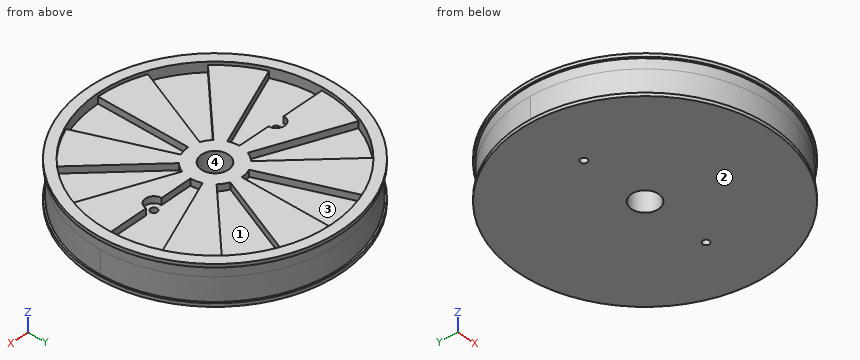
from build123d import *
from build123d.topology import SkipClean

# Parameters (mm, degrees)
CROQUIS1_R                 = 37.5
SALIENTE_EXTRUIR1_DEPTH    = 3.5
CROQUIS3_R                 = 38
SALIENTE_EXTRUIR2_DEPTH    = 1
SALIENTE_EXTRUIR4_START    = 1
CROQUIS5_R                 = 38
SALIENTE_EXTRUIR4_DEPTH    = 1
CROQUIS6_R                 = 4.05
CORTAR_EXTRUIR1_DEPTH      = 31
SALIENTE_EXTRUIR5_START    = 2
CROQUIS7_R                 = 8
CROQUIS7_R_2               = 4.05
SALIENTE_EXTRUIR5_DEPTH    = 2
SALIENTE_EXTRUIR7_START    = 2
SALIENTE_EXTRUIR7_DEPTH    = 2
SALIENTE_EXTRUIR8_START    = 3
CROQUIS10_R                = 38
CROQUIS10_R_2              = 35
SALIENTE_EXTRUIR8_DEPTH    = 3
CORTAR_EXTRUIR2_DEPTH      = 21
CORTAR_EXTRUIR2_DEPTH_BACK = 48
CROQUIS11_R                = 1
CROQUIS15_OUTSIDE_W        = 99.63
CROQUIS15_OUTSIDE_H        = 99.63
CROQUIS15_OUTSIDE_R        = 37.5
CORTAR_EXTRUIR6_DEPTH      = 10
CORTAR_EXTRUIR10_DEPTH     = 2


with BuildPart() as part:
    # Croquis1 → Saliente-Extruir1 (new, symmetric)
    with BuildSketch(Plane.XY):
        Circle(CROQUIS1_R)
    extrude(amount=SALIENTE_EXTRUIR1_DEPTH, both=True)

    # Croquis3 → Saliente-Extruir2 (add)
    with BuildSketch(Plane.XY.offset(3.5)):
        Circle(CROQUIS3_R)
    extrude(amount=SALIENTE_EXTRUIR2_DEPTH)

    # Croquis5 → Saliente-Extruir4 (add)
    with BuildSketch(Plane(origin=(0, 0, -3.5), x_dir=(-1, 0, 0), z_dir=(0, 0, -1)).offset(SALIENTE_EXTRUIR4_START)):
        with Locations(Location((0, 0, 0), (0, 0, 180))):
            Circle(CROQUIS5_R)
    extrude(amount=-SALIENTE_EXTRUIR4_DEPTH)

    # Croquis6 → Cortar-Extruir1 (cut)
    with BuildSketch(Plane.XY.offset(4.5)):
        Circle(CROQUIS6_R)
    extrude(amount=-CORTAR_EXTRUIR1_DEPTH, mode=Mode.SUBTRACT)

    # Croquis7 → Saliente-Extruir5 (add)
    with BuildSketch(Plane.XY.offset(4.5).offset(SALIENTE_EXTRUIR5_START)):
        Circle(CROQUIS7_R)
        Circle(CROQUIS7_R_2, mode=Mode.SUBTRACT)
    extrude(amount=-SALIENTE_EXTRUIR5_DEPTH)

    # Croquis9 → Saliente-Extruir7 (add)
    with BuildSketch(Plane.XY.offset(4.5).offset(SALIENTE_EXTRUIR7_START)):
        with BuildLine():
            Line((0, 35), (0, 8))
            ThreePointArc((0, 8), (1.560722576, 7.846282243), (3.061467459, 7.39103626))
            Line((3.061467459, 7.39103626), (13.393920133, 32.335783638))
            ThreePointArc((13.393920133, 32.335783638), (6.828161271, 34.327484814), (0, 35))
        make_face()
        with BuildLine():
            Line((-35, 0), (-8, 0))
            ThreePointArc((-8, 0), (-7.846282243, 1.560722576), (-7.39103626, 3.061467459))
            Line((-7.39103626, 3.061467459), (-32.335783638, 13.393920133))
            ThreePointArc((-32.335783638, 13.393920133), (-34.327484814, 6.828161271), (-35, 0))
        make_face()
        with BuildLine():
            Line((-24.748737342, 24.748737342), (-5.656854249, 5.656854249))
            ThreePointArc((-5.656854249, 5.656854249), (-4.444561864, 6.651756898), (-3.061467459, 7.39103626))
            Line((-3.061467459, 7.39103626), (-13.393920133, 32.335783638))
            ThreePointArc((-13.393920133, 32.335783638), (-19.444958156, 29.101436431), (-24.748737342, 24.748737342))
        make_face()
        with BuildLine():
            Line((24.748737342, 24.748737342), (5.656854249, 5.656854249))
            ThreePointArc((5.656854249, 5.656854249), (6.651756898, 4.444561864), (7.39103626, 3.061467459))
            Line((7.39103626, 3.061467459), (32.335783638, 13.393920133))
            ThreePointArc((32.335783638, 13.393920133), (29.101436431, 19.444958156), (24.748737342, 24.748737342))
        make_face()
        with BuildLine():
            Line((-5.656854249, -5.656854249), (-24.748737342, -24.748737342))
            ThreePointArc((-24.748737342, -24.748737342), (-29.101436431, -19.444958156), (-32.335783638, -13.393920133))
            Line((-32.335783638, -13.393920133), (-7.39103626, -3.061467459))
            ThreePointArc((-7.39103626, -3.061467459), (-6.651756898, -4.444561864), (-5.656854249, -5.656854249))
        make_face()
        with BuildLine():
            Line((8, 0), (35, 0))
            ThreePointArc((35, 0), (34.327484814, -6.828161271), (32.335783638, -13.393920133))
            Line((32.335783638, -13.393920133), (7.39103626, -3.061467459))
            ThreePointArc((7.39103626, -3.061467459), (7.846282243, -1.560722576), (8, 0))
        make_face()
        with BuildLine():
            Line((0, -8), (0, -35))
            ThreePointArc((0, -35), (-6.828161271, -34.327484814), (-13.393920133, -32.335783638))
            Line((-13.393920133, -32.335783638), (-3.061467459, -7.39103626))
            ThreePointArc((-3.061467459, -7.39103626), (-1.560722576, -7.846282243), (0, -8))
        make_face()
        with BuildLine():
            Line((3.061467459, -7.39103626), (13.393920133, -32.335783638))
            ThreePointArc((13.393920133, -32.335783638), (19.444958156, -29.101436431), (24.748737342, -24.748737342))
            Line((24.748737342, -24.748737342), (5.656854249, -5.656854249))
            ThreePointArc((5.656854249, -5.656854249), (4.444561864, -6.651756898), (3.061467459, -7.39103626))
        make_face()
    extrude(amount=-SALIENTE_EXTRUIR7_DEPTH)

    # Croquis10 → Saliente-Extruir8 (add)
    with BuildSketch(Plane.XY.offset(4.5).offset(SALIENTE_EXTRUIR8_START)):
        Circle(CROQUIS10_R)
        Circle(CROQUIS10_R_2, mode=Mode.SUBTRACT)
    extrude(amount=-SALIENTE_EXTRUIR8_DEPTH)

    # Croquis11 → Cortar-Extruir2 (cut, two sides: drawn at the far end of the back side and taken through both)
    with BuildSketch(Plane.XY.offset(6.5).offset(-CORTAR_EXTRUIR2_DEPTH_BACK)):
        with Locations(Location((-20, 0, 0), (0, 0, 180))):
            Circle(CROQUIS11_R)
        with Locations(Location((20, 0, 0), (0, 0, 180))):
            Circle(CROQUIS11_R)
    extrude(amount=CORTAR_EXTRUIR2_DEPTH + CORTAR_EXTRUIR2_DEPTH_BACK, mode=Mode.SUBTRACT)

    # Croquis15 outside → Cortar-Extruir6 (cut)
    with SkipClean():  # the faces are left unmerged after this step: merging them gives an invalid solid
        with BuildSketch(Plane.XY.offset(-3.5)):
            Rectangle(CROQUIS15_OUTSIDE_W, CROQUIS15_OUTSIDE_H)
            with Locations(Location((0, 0, 0), (0, 0, 180))):
                Circle(CROQUIS15_OUTSIDE_R, mode=Mode.SUBTRACT)
        extrude(amount=CORTAR_EXTRUIR6_DEPTH, mode=Mode.SUBTRACT)

    # Croquis17 → Cortar-Extruir10 (cut)
    with SkipClean():  # the faces are left unmerged after this step: merging them gives an invalid solid
        with BuildSketch(Plane.XY.offset(6.5)):
            with BuildLine():
                Line((22.5, 0), (21, 0))
                ThreePointArc((21, 0), (20, -1), (19, 0))
                Line((19, 0), (17.5, 0))
                ThreePointArc((17.5, 0), (20, -2.5), (22.5, 0))
            make_face()
            with BuildLine():
                Line((-21, 0), (-22.5, 0))
                ThreePointArc((-22.5, 0), (-20, 2.5), (-17.5, 0))
                Line((-17.5, 0), (-19, 0))
                ThreePointArc((-19, 0), (-20, 1), (-21, 0))
            make_face()
        extrude(amount=-CORTAR_EXTRUIR10_DEPTH, mode=Mode.SUBTRACT)


solid = part.part
Source: CAD feature listing. Evaluate the final solid. Frame: model axes, mm. Face numbers are marked on the shaded views. A direction names the side the tool comes from. Give positions to 0.01 mm unless a question says otherwise; leave off trailing zeros. Write each loop counter-clockwise with the first axis right and the second up, starting at its lowest first coordinate (ties: lowest second). Pieces come first, ordered by that corner, then holes. Notation, with made-up numbers: M 56,-36.75 L 90,-36.75 A26 ccw 90,-14.75 Z; hole C -6,44 d10. An arc over 180 degrees is marked long. Return JSON: item names as keys, results as strings. Group by question number.
1) Cut plane A-A, the plane x = -2. Output: boundary loops of the cut face in (y, z), then the cut area to 3 significant figures.
2) Cut plane C-C, the plane z = 5.5. Give the number of separate pieces and of enclosed holes in the cut face, then the cut area to 3 significant figures.
3) First-contact query: pin 1 Ø4 at (y, z) = (-24, -1) entering from -X; pin 2 Ø2 at (x, z) = (-10.5, 5) entering from -Y; pin 3 Ø3 at (x, y) = (19, -1.5) entering from +Z; pin 4 Ø1.6 at (x, y) = (20, 0) entering from -Z. Flat tips, straight axial feed; report the tip coordinate or a pass-through.
4) Set-up query: the marked faces 3 and 4. Return all of +Z, -Z, +X, -X, +Y, -Y with unobstructed straight access to the full face (end or side cutting, diameter ignored); none if empty.
5) Draft query along X for the marked faces 1 and 2. Return one class per face: released by +X, released by -X, zero draft, split by the parting line, or undercut.
6) Ray query, L1, parallel to Y at x = 0, z = 4; L2, parallel to Y at x = 15, z = 6; L3, parallel to Z at x = 13, y = 31. Return the intervals inside material, ascending.
7) Cut plane B-B, the plane y = 27.5. Output: boundary loops of the cut face in (x, z), then the cut area to 3 significant figures.
8) Cut plane D-D, the plane x = 27. Output: boundary loops of the cut face in (y, z), then the cut area to 3 significant figures.
Data:
{
 "1": {"outline": "M -37.95,-4.5 L -3.52,-4.5 L -3.52,6.5 L -34.94,6.5 L -34.94,7.5 L -37.95,7.5 L -37.95,6.5 L -37.45,6.5 L -37.45,-3.5 L -37.95,-3.5 Z; M 3.52,-4.5 L 37.95,-4.5 L 37.95,-3.5 L 37.45,-3.5 L 37.45,6.5 L 37.95,6.5 L 37.95,7.5 L 34.94,7.5 L 34.94,4.5 L 7.75,4.5 L 7.75,6.5 L 3.52,6.5 Z", "area": "699 mm²"},
 "2": {"separate pieces": "1", "enclosed holes": "9", "area": "2,520 mm²"},
 "3": {"pin 1": "stops at x = -30.37", "pin 2": "stops at y = -36.28", "pin 3": "stops at z = 6.5", "pin 4": "passes through"},
 "4": {"face 3": "+Z", "face 4": "+Z, -Z"},
 "5": {"face 1": "undercut", "face 2": "zero draft"},
 "6": {"L1": "y = -37.5 to -4.05, 4.05 to 37.5", "L2": "y = -34.37 to -15, -6.21 to 0, 6.21 to 15, 31.62 to 34.37", "L3": "z = -4.5 to 4.5"},
 "7": {"outline": "M -26.22,-4.5 L 26.22,-4.5 L 26.22,-3.5 L 25.5,-3.5 L 25.5,6.5 L 26.22,6.5 L 26.22,7.5 L 21.65,7.5 L 21.65,4.5 L 11.39,4.5 L 11.39,6.5 L 0,6.5 L 0,4.5 L -11.39,4.5 L -11.39,6.5 L -21.65,6.5 L -21.65,7.5 L -26.22,7.5 L -26.22,6.5 L -25.5,6.5 L -25.5,-3.5 L -26.22,-3.5 Z", "area": "528 mm²"},
 "8": {"outline": "M -26.74,-4.5 L 26.74,-4.5 L 26.74,-3.5 L 26.02,-3.5 L 26.02,6.5 L 26.74,6.5 L 26.74,7.5 L 22.27,7.5 L 22.27,6.5 L 11.18,6.5 L 11.18,4.5 L 0,4.5 L 0,6.5 L -11.18,6.5 L -11.18,4.5 L -22.27,4.5 L -22.27,7.5 L -26.74,7.5 L -26.74,6.5 L -26.02,6.5 L -26.02,-3.5 L -26.74,-3.5 Z", "area": "538 mm²"}
}
